from build123d import *

# Parameters (mm, degrees)
SKETCH1_R       = 45
EXTRUDE1_DEPTH  = 10
SKETCH2_W       = 10
SKETCH2_H       = 139
EXTRUDE2_DEPTH  = 82
CHAMFER1_SIZE   = 8
EXTRUDE3_START  = -5
EXTRUDE3_DEPTH  = 8
LPATTERN1_COUNT = 2
LPATTERN1_PITCH = 121


with BuildPart() as part:
    # Sketch1 → Extrude1 (new body)
    with BuildSketch(Plane(origin=(0, 0, 0), x_dir=(1, 0, 0), z_dir=(0, 1, 0))):
        Polygon((0, 69.5), (-68, 69.5), (-68, -69.5), (0, -69.5), (72, -69.5), (72, 69.5), align=None)
        with Locations(Location((0, 0, 0), (0, 0, 270))):
            Circle(SKETCH1_R, mode=Mode.SUBTRACT)
    extrude(amount=EXTRUDE1_DEPTH)

    # Sketch2 → Extrude2 (add)
    with BuildSketch(Plane(origin=(0, 10, 0), x_dir=(1, 0, 0), z_dir=(0, 1, 0))):
        with Locations((67, 0)):
            Rectangle(SKETCH2_W, SKETCH2_H)
    extrude(amount=EXTRUDE2_DEPTH)

    # Chamfer1
    chamfer1_edges = [part.edges().sort_by_distance(p)[0] for p in [
        (62, 92, 0),
    ]]
    chamfer(chamfer1_edges, length=CHAMFER1_SIZE)

    # Sketch3 → Extrude3 (add)
    with BuildSketch(Plane.XY.offset(69.5).offset(EXTRUDE3_START)):
        Polygon((12, 10), (62, 10), (62, 60), align=None)
    extrude3 = extrude(amount=-EXTRUDE3_DEPTH)

    # LPattern1: Extrude3 ×2
    with Locations(*[(0, 0, -i * LPATTERN1_PITCH) for i in range(1, LPATTERN1_COUNT)]):
        add(extrude3)


solid = part.part
Design review of the part built by this model. Coordinates are the model's own, in mm. A direction names the side the tool comes from. Coordinates: 2 decimals unless noted, no trailing zeros. Order: outer loops, then holes, each group sorted by start corner. A loop starts at its lowest first (then second) coordinate and runs counter-clockwise, first axis right, second up. Notation, with made-up numbers: (71, -29.5) - (94, -29.5) arc R26 ccw to (94, -12.5) - close; hole circle Ø7 at (75, 17). An arc over 180 degrees is marked (long way). Put each result on its own line as item: value.
1) Take a section at C-C, the plane y = 57.5. Give the boundary of the cut face in (x, z), and give its area (3 significant figures).
Response values:
outline: (59.5, -64.5) - (62, -64.5) - (62, -69.5) - (72, -69.5) - (72, 69.5) - (62, 69.5) - (62, 64.5) - (59.5, 64.5) - (59.5, 56.5) - (62, 56.5) - (62, -56.5) - (59.5, -56.5) - close
area: 1,430 mm²
2) The part is to be moulded in two halves that separate along X. For faces 5 (the face through (-68, 5, -1)), 6 (the face through (-17.235, 4.93, 41.569)), 7 (the face through (48, 24, -56.5)), 8 (the face through (72, 45, 1)), say which applies: released by +X, released by -X, zero draft, split by the parting line, or undercut.
Response values:
face 5: released by -X
face 6: undercut
face 7: zero draft
face 8: released by +X
3) Take a section at A-A, the plane x = 0. Give the boundary of the cut face in (y, z), and give its area (3 significant figures).
Response values:
outline: (0, -69.5) - (10, -69.5) - (10, -45) - (0, -45) - close; (0, 45) - (10, 45) - (10, 69.5) - (0, 69.5) - close
area: 490 mm²
4) Tool access review of faces 1 (the face through (17, 8, 69.5)), 2 (the face through (48, 24, 64.5)), 3 (the face through (48, 24, 56.5)), 4 (the face through (48, 24, -64.5)): name each direction out of +Z, -Z, +X, -X, +Y, -Y from which nothing blocks a thin tool from reaching the whole face with its end or side.
Response values:
face 1: +Z, +X, -X, +Y, -Y
face 2: +Z, -X, +Y
face 3: -X, +Y
face 4: -Z, -X, +Y
5) Take a section at D-D, the plane z = -25.5. Give the boundary of the cut face in (x, y).
Response values:
outline: (-68, 0) - (-37.08, 0) - (-37.08, 10) - (-68, 10) - close; (37.08, 0) - (72, 0) - (72, 92) - (70, 92) - (62, 84) - (62, 10) - (37.08, 10) - close
6) Insertion check: P1, Ø25, axis at x = 30, y = 36.5, coming from the +Z side. The pin has a flat end and moves straight along its axis. Give the tip position at first contact, or say it passes through.
Response values:
P1: stops at z = 64.5
7) Take a section at B-B, the plane z = 0. Give the boundary of the cut face in (x, y).
Response values:
outline: (-68, 0) - (-45, 0) - (-45, 10) - (-68, 10) - close; (45, 0) - (72, 0) - (72, 92) - (70, 92) - (62, 84) - (62, 10) - (45, 10) - close
8) Wall thickness on L1, parallel to Z at x = 47, y = 19; L2, parallel to X at y = 5, z = 0; L3, parallel to Y at x = 14.5, z = 44.5: over which ranges is each line inside the solid? List them lowest first. Write a range as from..to.
Response values:
L1: z = -64.5..-56.5, 56.5..64.5
L2: x = -68..-45, 45..72
L3: y = 0..10
